Part model, mm, in its own coordinate system. A direction names the side the tool comes from. Round coordinates to 2 decimals unless told otherwise and drop trailing zeros. Write each loop counter-clockwise with the first axis right and the second up, starting at its lowest first coordinate (ties: lowest second). Pieces come first, ordered by that corner, then holes.
```python
from build123d import *

# Parameters (mm, degrees)
BOSS_EXTRUDE3_DEPTH = 2
BOSS_EXTRUDE6_DEPTH = 22.5
SKETCH10_R          = 1.5
SKETCH10_R_2        = 3.5
CUT_EXTRUDE3_DEPTH  = 99.360002033
RIB6_START          = -3
RIB6_DEPTH          = 3
RIB7_START          = -1.5
RIB7_DEPTH          = 3
RIB8_DEPTH          = 3
SKETCH22_R          = 1.5
CUT_EXTRUDE5_DEPTH  = 102.088772868
SKETCH23_R          = 1.5
CUT_EXTRUDE6_DEPTH  = 102.088772868
SKETCH24_R          = 1.5
CUT_EXTRUDE7_DEPTH  = 10
SKETCH25_R          = 1.5
CUT_EXTRUDE8_DEPTH  = 10


# Read off the part's stored shape, not the designer's step: Rib6, Rib7, Rib8
with BuildPart() as part:
    # vlak basis → Boss-Extrude3 (new body)
    with BuildSketch(Plane(origin=(0, 0, 0), x_dir=(1, 0, 0), z_dir=(0, 1, 0))):
        with BuildLine():
            Line((-46.3, -61.5), (-46.3, -75))
            Line((-46.3, -75), (-14, -75))
            Line((-14, -75), (-14, -80))
            ThreePointArc((-14, -80), (-11.949747468, -84.949747468), (-7, -87))
            ThreePointArc((-7, -87), (-2.050252532, -84.949747468), (0, -80))
            Line((0, -80), (0, 0))
            Line((0, 0), (-14.3, 0))
            ThreePointArc((-14.3, 0), (-21.3, 7), (-28.3, 0))
            Line((-28.3, 0), (-28.3, -61.5))
            Line((-28.3, -61.5), (-46.3, -61.5))
        make_face()
    extrude(amount=BOSS_EXTRUDE3_DEPTH)

    # Sketch8 → Boss-Extrude6 (add)
    with BuildSketch(Plane(origin=(0, 2, 0), x_dir=(1, 0, 0), z_dir=(0, 1, 0))):
        Polygon((-16.5, -7), (-16.5, -15), (-9.5, -15), (-9.5, -54), (-7.5, -54), (-7.5, -7), align=None)
    extrude(amount=BOSS_EXTRUDE6_DEPTH)

    # Sketch10 → Cut-Extrude3 (cut, through all)
    with BuildSketch(Plane(origin=(-7.5, 0, 0), x_dir=(0, 0, -1), z_dir=(1, 0, 0))):
        with Locations((-46.6, 22)):
            Circle(SKETCH10_R)
        with Locations((-46.6, 4.5)):
            Circle(SKETCH10_R)
        with Locations((-26.2, 13.25)):
            Circle(SKETCH10_R_2)
        with Locations((-12.6, 13.25)):
            Circle(SKETCH10_R)
    extrude(amount=-CUT_EXTRUDE3_DEPTH, mode=Mode.SUBTRACT)

    # Rib6 outline → Rib6 (add)
    with BuildSketch(Plane.XY.offset(54).offset(RIB6_START)):
        Polygon((-7.5, 2), (0, 2), (-7.5, 24.5), align=None)
    extrude(amount=RIB6_DEPTH)

    # Rib7 outline → Rib7 (add)
    with BuildSketch(Plane.XY.offset(38).offset(RIB7_START)):
        Polygon((-7.5, 2), (0, 2), (-7.5, 24.5), align=None)
    extrude(amount=RIB7_DEPTH)

    # Rib8 outline → Rib8 (add)
    with BuildSketch(Plane.XY.offset(17)):
        Polygon((-7.5, 2), (0, 2), (-7.5, 24.5), align=None)
    extrude(amount=RIB8_DEPTH)

    # Sketch22 → Cut-Extrude5 (cut, through all)
    with BuildSketch(Plane(origin=(0, 2, 0), x_dir=(1, 0, 0), z_dir=(0, 1, 0))):
        with Locations(Location((-21.3, 0, 0), (0, 0, 270))):
            Circle(SKETCH22_R)
    extrude(amount=-CUT_EXTRUDE5_DEPTH, mode=Mode.SUBTRACT)

    # Sketch23 → Cut-Extrude6 (cut, through all)
    with BuildSketch(Plane(origin=(0, 2, 0), x_dir=(1, 0, 0), z_dir=(0, 1, 0))):
        with Locations(Location((-7, -80, 0), (0, 0, 270))):
            Circle(SKETCH23_R)
    extrude(amount=-CUT_EXTRUDE6_DEPTH, mode=Mode.SUBTRACT)

    # Sketch24 → Cut-Extrude7 (cut)
    with BuildSketch(Plane(origin=(0, 2, 0), x_dir=(1, 0, 0), z_dir=(0, 1, 0))):
        with Locations(Location((-42.3, -68.25, 0), (0, 0, 270))):
            Circle(SKETCH24_R)
    extrude(amount=-CUT_EXTRUDE7_DEPTH, mode=Mode.SUBTRACT)

    # Sketch25 → Cut-Extrude8 (cut)
    with BuildSketch(Plane(origin=(0, 2, 0), x_dir=(1, 0, 0), z_dir=(0, 1, 0))):
        with Locations(Location((-4, -4, 0), (0, 0, 270))):
            Circle(SKETCH25_R)
    extrude(amount=-CUT_EXTRUDE8_DEPTH, mode=Mode.SUBTRACT)


with BuildPart() as body_2:
    # Mirror1: mirrored copy
    add(part.part.mirror(Plane(origin=(0, 2, 80), x_dir=(0, 0, 1), z_dir=(-1, 0, 0))))


solid = body_2.part
```
Q1. Wall check: L1, parallel to Y at x = 9.15, z = 46.6; L2, parallel to X at y = 0.9, z = 4; L3, parallel to Y at x = 8, z = 12.5. Give the ranges that are in metal, low to high.
Values follow:
L1: y = 0 to 3, 6 to 20.5, 23.5 to 24.5
L2: x = 0 to 2.5, 5.5 to 28.3
L3: y = 0 to 11.75, 14.75 to 24.5
Q2. Mould opens along X. For faces 5 (the flat face through (7.5, 13, 45)), 6 (the flat face through (9, 24.5, 20)), 7 (the cylindrical face through (3.55, 1.01, 5.43)), 8 (the flat face through (28.3, 1, 30)) say: +X half, -X half, draft (parallel to the pull), parting line (faces both ways), or undercut.
Values follow:
face 5: -X half
face 6: draft
face 7: undercut
face 8: +X half
Q3. Cut at C-C on z = 26.2. Write the cut outline in (x, y).
Values follow:
outline: (0, 0) - (28.3, 0) - (28.3, 2) - (9.5, 2) - (9.5, 9.75) - (7.5, 9.75) - (7.5, 2) - (0, 2) - close; (7.5, 16.75) - (9.5, 16.75) - (9.5, 24.5) - (7.5, 24.5) - close
Q4. Drop flat-ended pins along their axis: pin 1 (6 mm diameter, centred on x = 3.5, y = 9, fed in from +Z); pin 2 (4 mm diameter, centred on x = 2, y = 10, fed in from -Z); pin 3 (6 mm diameter, centred on x = 5, z = 14.5, fed in from -Y); pin 4 (5 mm diameter, centred on y = 10, z = 13.5, fed in from -X). Give the stop position or say it passes through.
Values follow:
pin 1: stops at z = 54
pin 2: stops at z = 17
pin 3: stops at y = 0
pin 4: stops at x = 7.5
Q5. Cut at A-A on x = 42.3. Write the cut outline in (y, z), plus the area to 3 significant figures.
Values follow:
outline: (0, 61.5) - (2, 61.5) - (2, 66.75) - (0, 66.75) - close; (0, 69.75) - (2, 69.75) - (2, 75) - (0, 75) - close
area: 21.0 mm2
Q6. Cut at B-B on z = 52. Write the cut outline in (x, y).
Values follow:
outline: (0, 0) - (28.3, 0) - (28.3, 2) - (9.5, 2) - (9.5, 24.5) - (7.5, 24.5) - (0, 2) - close
Q7. Cut at D-D on y = 8.5. Write the cut outline in (x, z).
Values follow:
outline: (2.17, 17) - (7.5, 17) - (7.5, 7) - (16.5, 7) - (16.5, 15) - (9.5, 15) - (9.5, 54) - (2.17, 54) - (2.17, 51) - (7.5, 51) - (7.5, 39.5) - (2.17, 39.5) - (2.17, 36.5) - (7.5, 36.5) - (7.5, 20) - (2.17, 20) - close
Q8. Which spindle directions (+Z, -Z, +X, -X, +Y, -Y) get a long thin tool onto all of the face, cutting with end or side? Do faces 1 (the flat face through (7.5, 13, 10)), 2 (the flat face through (16.5, 13.1, 10.9)), 3 (the flat face through (12, 13, 7)), 4 (the flat face through (37, 1, 61.5)). Say none if no direction does.
Values follow:
face 1: -Z, -X, +Y
face 2: +Z, -Z, +X, +Y
face 3: -Z, +X, -X, +Y
face 4: -Z, +X, +Y, -Y
